Here's how the part is built. I have some questions about the finished solid (model axes, mm). A direction names the side the tool comes from. Round coordinates to 2 decimals unless told otherwise and drop trailing zeros. Loops run counter-clockwise (first coordinate to the right, second up) from the corner with the lowest first, then second, coordinate; pieces in that order, holes last. Notation, with made-up numbers: M 54.5,42.5 L 89.5,42.5 A29 ccw 89.5,72.5 Z; hole C 81,51.25 d2. An arc over 180 degrees is marked long. Answer as a JSON object with one key per item and string values.
from build123d import *

# Parameters (mm, degrees)
ESQUISSE1_R        = 22.5
BOSS_EXTRU_1_DEPTH = 24
ESQUISSE1_4_R      = 35.125
ESQUISSE1_4_R_2    = 22.5
BOSS_EXTRU_2_DEPTH = 28
CONG_1_R           = 1


with BuildPart() as part:
    # Esquisse1 → Boss.-Extru.1 (new body)
    with BuildSketch(Plane.XY):
        Circle(ESQUISSE1_R)
    extrude(amount=BOSS_EXTRU_1_DEPTH)

    # Esquisse1<4> → Boss.-Extru.2 (add)
    with BuildSketch(Plane.XY):
        Circle(ESQUISSE1_4_R)
        Circle(ESQUISSE1_4_R_2, mode=Mode.SUBTRACT)
    extrude(amount=BOSS_EXTRU_2_DEPTH)

    # Congé1
    cong_1_edges = [part.edges().sort_by_distance(p)[0] for p in [
        (-35.125, 0, 28),
        (-35.125, 0, 0),
        (-22.5, 0, 24),
        (-22.5, 0, 28),
    ]]
    fillet(cong_1_edges, radius=CONG_1_R)


solid = part.part
Item 1: I want a section at C-C, the plane z = 19.5. Please give me the cut outline in (x, y) (3 decimals).
Resolved:
{"outline": "C 0,0 d70.25"}
Item 2: On a 3-axis mill with a long thin cutter (end or side, diameter ignored), from which of +Z, -Z, +X, -X, +Y, -Y can I reach the whole of each face in a straight line? I mean faces 1 (the face through (10.382, -19.961, 25.986)), 2 (the face through (0, 0, 0)). Say none if no direction works.
Resolved:
{"face 1": "+Z", "face 2": "-Z, +X, -X, +Y, -Y"}
Item 3: Please list where these lines run through material, in increasing order: probe 1 along Y at (x, z) = (0, 26.55) (3 decimals); probe 2 along Z at (x, y) = (0, -5); probe 3 along X at (y, z) = (1, 26). Write a range as from..to.
Resolved:
{"probe 1": "-35.125..-22.5, 22.5..35.125", "probe 2": "0..24", "probe 3": "-35.11..-22.48, 22.48..35.11"}
Item 4: If we mould it in two halves opening along Y, with no side actions, what happens to faces 3 (the face through (0, 0, 24)), 4 (the face through (-8.1, -22.3, 28)), 5 (the face through (-27.874, -21.373, 13.818))? For each: pulls with the +Y half, pulls with the -Y half, needs draft (parallel to the pull), parting line crosses it, or undercut.
Resolved:
{"face 3": "undercut", "face 4": "needs draft", "face 5": "parting line crosses it"}
Item 5: I want a section at A-A, the plane y = 0. Please give me the cut outline in (x, z) (3 decimals).
Resolved:
{"outline": "M -35.125,1 A1 ccw -34.125,0 L 34.125,0 A1 ccw 35.125,1 L 35.125,27 A1 ccw 34.125,28 L 23.5,28 A1 ccw 22.5,27 L 22.5,25 A1 cw 21.5,24 L -21.5,24 A1 cw -22.5,25 L -22.5,27 A1 ccw -23.5,28 L -34.125,28 A1 ccw -35.125,27 Z"}
Item 6: I'm going to push flat-ended pins straight in: pin 1 Ø21.5 at (x, y) = (-6.5, 6) entering from +Z; pin 2 Ø1.5 at (y, z) = (-16.5, 13) entering from +X; pin 3 Ø1 at (y, z) = (24.5, 23.5) entering from +X. Where does each tip first touch, or does it pass through?
Resolved:
{"pin 1": "z = 24", "pin 2": "x = 31.4", "pin 3": "x = 25.65"}
